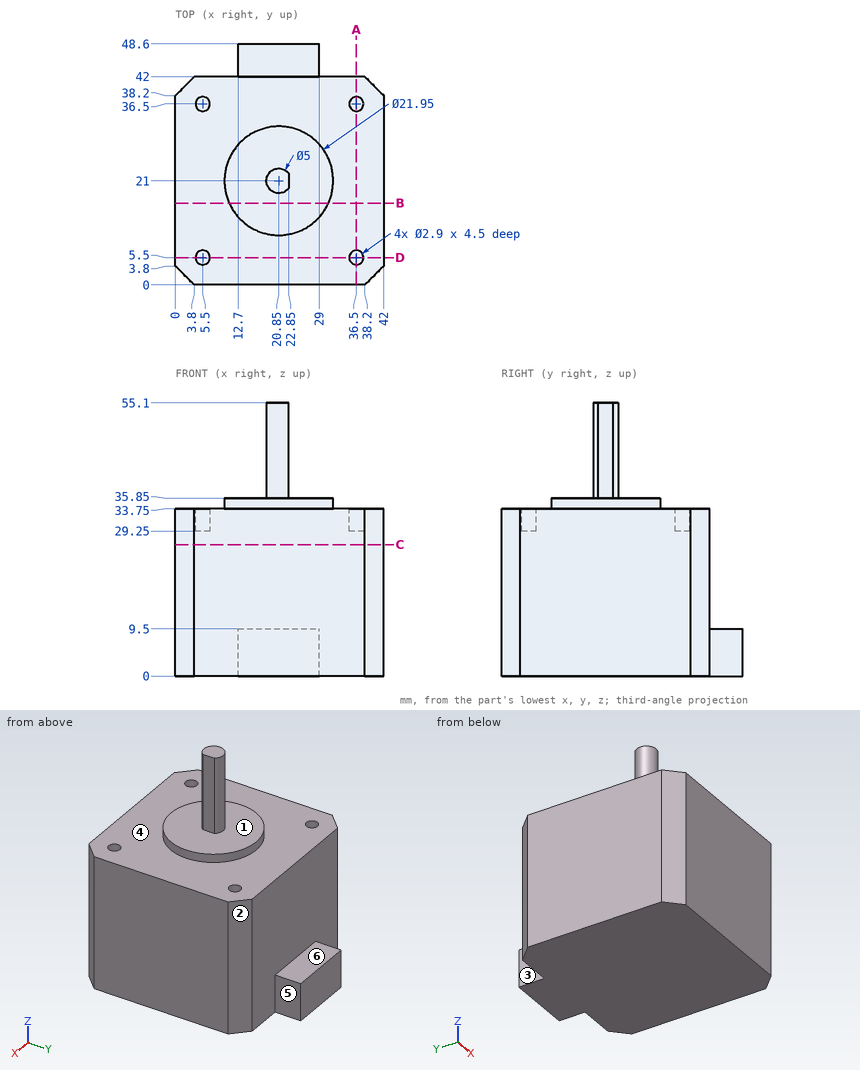
For this review, use the dimensioned drawing (mm, ordinates from the lowest corner) and the shaded views. A direction names the side the tool comes from. Give positions to 0.01 mm unless a question says otherwise; leave off trailing zeros. Order: outer loops, then holes, each group sorted by start corner. A loop starts at its lowest first (then second) coordinate and runs counter-clockwise, first axis right, second up.
1) Take a section at A-A (x = 36.5). Give the boundary of the cut face in (y, z).
2) Take a section at B-B (y = 16.5). Give the boundary of the cut face in (x, z).
3) Take a section at C-C (z = 26.5). Give the boundary of the cut face in (x, y).
4) For the marked faces 4, 5 and 6, list the 3-axis set-ups (+Z, -Z, +X, -X, +Y, -Y) from which the entire face can be reached by the end or side of a thin tool; tool diameter is ignored.
5) Wall thickness on line 1 (Y direction, x = 5.5, z = 31.4); line 2 (X direction, y = 36, z = 31); line 3 (Z direction, x = 18, y = 16): over which ranges is each line inside the solid? List them lowest first.
6) Insertion check: pin 1 (7.5 mm diameter, centred on y = 44, z = 3, fed in from -X); pin 2 (1.5 mm diameter, centred on y = 21, z = 47, fed in from +X); pin 3 (12 mm diameter, centred on x = 5.5, z = 32, fed in from +Y). Each pin has a flat end and moves straight along its axis. Give the tip position at first contact, or say it passes through.
7) The part is to be moulded in two halves that separate along X. For the marked faces 1, 2 and 3, say which applies: released by +X, released by -X, zero draft, split by the parting line, or undercut.
Derived:
1. outline: (0, 0) - (42, 0) - (42, 33.75) - (37.95, 33.75) - (37.95, 29.25) - (35.05, 29.25) - (35.05, 33.75) - (6.95, 33.75) - (6.95, 29.25) - (4.05, 29.25) - (4.05, 33.75) - (0, 33.75) - close
2. outline: (0, 0) - (42, 0) - (42, 33.75) - (30.86, 33.75) - (30.86, 35.85) - (10.84, 35.85) - (10.84, 33.75) - (0, 33.75) - close
3. outline: (0, 3.8) - (3.8, 0) - (38.2, 0) - (42, 3.8) - (42, 38.2) - (38.2, 42) - (3.8, 42) - (0, 38.2) - close
4. face 4: +Z
4. face 5: +Z, -Z, +X, +Y
4. face 6: +Z, +X, -X, +Y
5. line 1: y = 0 to 4.05, 6.95 to 35.05, 37.95 to 42
5. line 2: x = 0 to 4.14, 6.86 to 35.14, 37.86 to 42
5. line 3: z = 0 to 35.85
6. pin 1: stops at x = 2.05
6. pin 2: stops at x = 22.85
6. pin 3: stops at y = 42
7. face 1: zero draft
7. face 2: released by +X
7. face 3: released by -X
